```python
from build123d import *

# Parameters (mm, degrees)
SKETCH_1_R               = 6
EXTRUDE_1_DEPTH          = 45.7
CUT_EXTRUDE_START        = -12
CUT_EXTRUDE_1_DEPTH      = 12
SKETCH_3_OUTSIDE_W       = 23.75
SKETCH_3_OUTSIDE_H       = 23.75
SKETCH_3_OUTSIDE_R       = 4
CUT_EXTRUDE_2_DEPTH      = 31.2
SKETCH_4_OUTSIDE_W       = 23.75
SKETCH_4_OUTSIDE_H       = 23.75
SKETCH_4_OUTSIDE_R       = 3
CUT_EXTRUDE_3_DEPTH      = 13.3
CUT_EXTRUDE_4_DEPTH      = 47.481071416
CUT_EXTRUDE_4_DEPTH_BACK = 47.481071416
SKETCH_5_R               = 1.3


with BuildPart() as part:
    # ｽｹｯﾁ1 → ﾎﾞｽ - 押し出し1 (new body)
    with BuildSketch(Plane(origin=(0, 0, 0), x_dir=(0, 0, -1), z_dir=(1, 0, 0))):
        with Locations(Location((0, 0, 0), (0, 0, 180))):
            Circle(SKETCH_1_R)
    extrude(amount=EXTRUDE_1_DEPTH)

    # ｽｹｯﾁ2 → ｶｯﾄ - 押し出し1 (cut)
    with BuildSketch(Plane(origin=(45.7, 0, 0), x_dir=(0, 0, -1), z_dir=(1, 0, 0)).offset(CUT_EXTRUDE_START)):
        with BuildLine():
            ThreePointArc((5.454356057, 2.5), (0, 6), (-5.454356057, 2.5))
            Line((-5.454356057, 2.5), (-1.658312395, 2.5))
            ThreePointArc((-1.658312395, 2.5), (0, -3), (1.658312395, 2.5))
            Line((1.658312395, 2.5), (5.454356057, 2.5))
        make_face()
    extrude(amount=CUT_EXTRUDE_1_DEPTH, mode=Mode.SUBTRACT)

    # ｽｹｯﾁ3 outside → ｶｯﾄ - 押し出し2 (cut)
    with BuildSketch(Plane.ZY):
        Rectangle(SKETCH_3_OUTSIDE_W, SKETCH_3_OUTSIDE_H)
        Circle(SKETCH_3_OUTSIDE_R, mode=Mode.SUBTRACT)
    extrude(amount=-CUT_EXTRUDE_2_DEPTH, mode=Mode.SUBTRACT)

    # ｽｹｯﾁ4 outside → ｶｯﾄ - 押し出し3 (cut)
    with BuildSketch(Plane.ZY):
        Rectangle(SKETCH_4_OUTSIDE_W, SKETCH_4_OUTSIDE_H)
        Circle(SKETCH_4_OUTSIDE_R, mode=Mode.SUBTRACT)
    extrude(amount=-CUT_EXTRUDE_3_DEPTH, mode=Mode.SUBTRACT)

    # ｽｹｯﾁ5 → ｶｯﾄ - 押し出し4 (cut, two sides: drawn at the far end of the back side and taken through both)
    with BuildSketch(Plane(origin=(0, 0, 0), x_dir=(1, 0, 0), z_dir=(0, 1, 0)).offset(-CUT_EXTRUDE_4_DEPTH_BACK)):
        with Locations(Location((26.2, 0, 0), (0, 0, 270))):
            Circle(SKETCH_5_R)
    extrude(amount=CUT_EXTRUDE_4_DEPTH + CUT_EXTRUDE_4_DEPTH_BACK, mode=Mode.SUBTRACT)


solid = part.part
```
Geometry check sheet. Reference: the model listing, model coordinates, mm. A direction names the side the tool comes from. Round coordinates to 2 decimals unless told otherwise and drop trailing zeros. Order: outer loops, then holes, each group sorted by start corner. A loop starts at its lowest first (then second) coordinate and runs counter-clockwise, first axis right, second up. Notation, with made-up numbers: (1.5, -37) - (31.5, -37) arc R13 cw to (31.5, -33) - close; hole circle Ø2 at (-5, -10). An arc over 180 degrees is marked (long way). Use a Markdown table: item, result. Add a question column.
(1) Sectioned sample at B-B, the plane y = 0. Enter the section's corners in (x, z).
(2) Material ranges on line 1 along X through (y, z) = (2, 0); line 2 along Y through (x, z) = (40.5, 0); line 3 along X through (y, z) = (2.25, 3), recorded low to high. Write a range as [from, to].
(3) Sectioned sample at D-D, the plane x = 24. Enter the section's corners in (y, z), and give its area (3 significant figures).
(4) Sectioned sample at C-C, the plane z = -3.5. Enter the section's corners in (x, y).
(5) Tool access check on faces 4 (the flat face through (40, 2.5, 4)), 5 (the cylindrical face through (7, 0, -3)), 6 (the cylindrical face through (40, -3, 0)), 7 (the flat face through (45.7, -3, 1)). Record the directions out of +Z, -Z, +X, -X, +Y, -Y that give a thin tool (end or side, any length) a straight path to the whole face; none if there is none.
(6) Sectioned sample at A-A, the plane z = 0. Enter the section's corners in (x, y), and give its area (3 significant figures).
(7) Depth check by flat-ended pin: pin 1 (4 mm diameter, centred on x = 40, z = -4, fed in from +Y); pin 2 (3 mm diameter, centred on x = 5.5, y = 2, fed in from -Z); pin 3 (6 mm diameter, centred on x = 37.5, z = 3.5, fed in from -Y); pin 4 (2 mm diameter, centred on x = 26.2, z = 0, fed in from +Y). Enter the tip coordinate at first touch or a pass-through.
(8) Release check for a two-part mould opening along Z. For faces 1 (the flat face through (40, 2.5, -4)), 2 (the cylindrical face through (22.125, -1.532, 3.695)), 3 (the cylindrical face through (27.49, -0.06, -0.17)) record: pulls with the +Z half, pulls with the -Z half, needs draft (parallel to the pull), parting line crosses it, or undercut.
Answers below:
| question | item | result |
|---|---|---|
| 1 | outline | (0, -3) - (13.3, -3) - (13.3, -4) - (31.2, -4) - (31.2, -6) - (45.7, -6) - (45.7, -3) - (33.7, -3) - (33.7, 3) - (45.7, 3) - (45.7, 6) - (31.2, 6) - (31.2, 4) - (13.3, 4) - (13.3, 3) - (0, 3) - close; hole circle Ø2.6 at (26.2, 0) |
| 2 | line 1 | [0, 24.9], [27.5, 33.7] |
| 2 | line 2 | [-6, -3] |
| 2 | line 3 | [13.3, 45.7] |
| 3 | outline | circle Ø8 at (0, 0) |
| 3 | area | 50.3 mm² |
| 4 | outline | (13.3, -1.94) - (31.2, -1.94) - (31.2, -4.87) - (45.7, -4.87) - (45.7, 2.5) - (33.7, 2.5) - (33.7, 4.87) - (31.2, 4.87) - (31.2, 1.94) - (13.3, 1.94) - close |
| 5 | face 4 | +Z, -Z, +X, +Y |
| 5 | face 5 | -X |
| 5 | face 6 | +X |
| 5 | face 7 | +Z, -Z, +X, +Y, -Y |
| 6 | outline | (0, -3) - (13.3, -3) - (13.3, -4) - (24.9, -4) - (24.9, 4) - (13.3, 4) - (13.3, 3) - (0, 3) - close; (27.5, -4) - (31.2, -4) - (31.2, -6) - (45.7, -6) - (45.7, -3) - (33.7, -3) - (33.7, 6) - (31.2, 6) - (31.2, 4) - (27.5, 4) - close |
| 6 | area | 268 mm² |
| 7 | pin 1 | y = 2.5 |
| 7 | pin 2 | z = -2.96 |
| 7 | pin 3 | y = -5.98 |
| 7 | pin 4 | through |
| 8 | face 1 | needs draft |
| 8 | face 2 | parting line crosses it |
| 8 | face 3 | undercut |
